Design review of the part built by this model. Coordinates are the model's own, in mm. A direction names the side the tool comes from. Give positions to 0.01 mm unless a question says otherwise; leave off trailing zeros. Write each loop counter-clockwise with the first axis right and the second up, starting at its lowest first coordinate (ties: lowest second). Pieces come first, ordered by that corner, then holes.
```python
from build123d import *

# Parameters (mm, degrees)
SKETCH1_R           = 19
BOSS_EXTRUDE1_DEPTH = 3
BOSS_EXTRUDE2_DEPTH = 13


with BuildPart() as part:
    # Sketch1 → Boss-Extrude1 (new body)
    with BuildSketch(Plane(origin=(0, 0, 0), x_dir=(1, 0, 0), z_dir=(0, 1, 0))):
        with Locations(Location((0, 0, 0), (0, 0, 270))):  # turned: the seam where the file's is
            Circle(SKETCH1_R)
    extrude(amount=BOSS_EXTRUDE1_DEPTH)

    # Sketch2 → Boss-Extrude2 (add)
    with BuildSketch(Plane(origin=(0, 3, 0), x_dir=(1, 0, 0), z_dir=(0, 1, 0))):
        with BuildLine():
            Line((-8, -3), (-8, 3))
            ThreePointArc((-8, 3), (0, 11), (8, 3))
            Line((8, 3), (8, -3))
            ThreePointArc((8, -3), (0, -11), (-8, -3))
        make_face()
    extrude(amount=BOSS_EXTRUDE2_DEPTH)


solid = part.part
```
(1) Consider section A-A, the plane x = 0. Give the boundary of the cut face in (y, z).
Resolved:
outline: (0, -19) - (3, -19) - (3, -11) - (16, -11) - (16, 11) - (3, 11) - (3, 19) - (0, 19) - close
(2) Consider section B-B, the plane z = 0. Give the boundary of the cut face in (x, y).
Resolved:
outline: (-19, 0) - (19, 0) - (19, 3) - (8, 3) - (8, 16) - (-8, 16) - (-8, 3) - (-19, 3) - close
(3) To check wall thickness, follow L1, parallel to Y at x = -16.5, z = -8; L2, parallel to Z at x = -0.5, y = 1.75; L3, parallel to X at y = 8, z = 2. State the ranges of each line that lie inside material, in increasing order.
Resolved:
L1: y = 0 to 3
L2: z = -18.99 to 18.99
L3: x = -8 to 8
(4) Tool access review of faces 1 (the face through (8, 9, 0)), 2 (the face through (-8.2, 3, -0.3)), 3 (the face through (-8, 9, 0)), 4 (the face through (0, 9, -11)), 5 (the face through (0, 9, 11)): name each direction out of +Z, -Z, +X, -X, +Y, -Y from which nothing blocks a thin tool from reaching the whole face with its end or side.
Resolved:
face 1: +Z, -Z, +X, +Y
face 2: +Y
face 3: +Z, -Z, -X, +Y
face 4: -Z, +Y
face 5: +Z, +Y
(5) Clearance check with flat-ended pins moving along their axes: P1, Ø4, axis at x = -1.5, y = 6, coming from the -Z side; P2, Ø1, axis at x = -14, z = -3, coming from the +Y side; P3, Ø5, axis at y = 9.5, z = -0.5, coming from the -X side. State where each tip first meets the part, or that it passes through.
Resolved:
P1: stops at z = -11
P2: stops at y = 3
P3: stops at x = -8
(6) Consider section D-D, the plane y = 5.5. Give the boundary of the cut face in (x, z), then the cut area to 3 significant figures.
Resolved:
outline: (-8, -3) arc R8 ccw to (8, -3) - (8, 3) arc R8 ccw to (-8, 3) - close
area: 297 mm2
(7) Consider section C-C, the plane y = 2.25. Give the boundary of the cut face in (x, z).
Resolved:
outline: circle Ø38 at (0, 0)
